The listing builds one solid part. Answer for the finished solid, in the listing's coordinates (mm). A direction names the side the tool comes from. Give positions to 0.01 mm unless a question says otherwise; leave off trailing zeros. Write each loop counter-clockwise with the first axis right and the second up, starting at its lowest first coordinate (ties: lowest second). Pieces come first, ordered by that corner, then holes. Notation, with made-up numbers: M 59.25,-9 L 93.25,-9 A5 cw 93.25,-4 Z; hole C 89.25,5.5 d8. An arc over 180 degrees is marked long. Answer as a JSON object with one key per item and string values.
```python
from build123d import *

# Parameters (mm, degrees)
SKETCH1_R           = 26.25
BOSS_EXTRUDE1_DEPTH = 133.5
SKETCH3_R           = 26.25
CUT_EXTRUDE1_DEPTH  = 232.63225164
CUT_EXTRUDE2_START  = -210
CUT_EXTRUDE2_DEPTH  = 105
FILLET1_R           = 20


with BuildPart() as part:
    # Sketch1 → Boss-Extrude1 (new body)
    with BuildSketch(Plane.XY):
        with BuildLine():
            Line((-52.5, 0), (-52.5, -157.5))
            Line((-52.5, -157.5), (52.5, -157.5))
            Line((52.5, -157.5), (52.5, 0))
            ThreePointArc((52.5, 0), (0, 52.5), (-52.5, 0))
        make_face()
        Circle(SKETCH1_R, mode=Mode.SUBTRACT)
    extrude(amount=BOSS_EXTRUDE1_DEPTH)

    # Sketch3 → Cut-Extrude1 (cut, through all)
    with BuildSketch(Plane.ZY.offset(52.5)):
        with Locations(Location((66.75, -105, 0), (0, 0, 270))):
            Circle(SKETCH3_R)
    extrude(amount=-CUT_EXTRUDE1_DEPTH, mode=Mode.SUBTRACT)

    # Sketch6 → Cut-Extrude2 (cut)
    with BuildSketch(Plane.XZ.offset(157.5).offset(CUT_EXTRUDE2_START)):
        Polygon((-52.5, 66.75), (-52.5, 44.5), (52.5, 44.5), (52.5, 89), (-52.5, 89), align=None)
    extrude(amount=CUT_EXTRUDE2_DEPTH, mode=Mode.SUBTRACT)

    # Fillet1
    fillet1_edges = [part.edges().sort_by_distance(p)[0] for p in [
        (0, -157.5, 133.5),
        (0, -157.5, 0),
    ]]
    fillet(fillet1_edges, radius=FILLET1_R)


solid = part.part
```
1. A cutting plane is placed at D-D, the plane z = 29. Give the vertices of the cut face in (x, y).
Verdict:
{"outline": "M -52.5,-157.5 L 52.5,-157.5 L 52.5,0 A52.5 ccw -52.5,0 Z; hole C 0,0 d52.5"}
2. A flat-ended cylindrical pin translates along its axis: pin 1 (6 mm diameter, centred on x = 19.5, z = 83, fed in from +Y). Find the tip coordinate at first contact, or state that the pin passes through.
Verdict:
{"pin 1": "stops at y = -52.5"}
3. The mould has two halves that part along Y. Classify faces 3 (the cylindrical face through (-1, -84, 51)), 4 (the cylindrical face through (0.735, -151.486, 127.797)), 5 (the flat face through (-1, -52.5, 67)): released by +Y, released by -Y, zero draft, split by the parting line, or undercut.
Verdict:
{"face 3": "undercut", "face 4": "released by -Y", "face 5": "released by +Y"}
4. A cutting plane is placed at B-B, the plane y = -105. Give the vertices of the cut face in (x, z), plus the area to 4 significant figures.
Verdict:
{"outline": "M -52.5,0 L 52.5,0 L 52.5,40.5 L -52.5,40.5 Z; M -52.5,93 L 52.5,93 L 52.5,133.5 L -52.5,133.5 Z", "area": "8,505 mm2"}
5. Consider line 1 along Y through (x, z) = (0, 105); line 2 along Z through (x, y) = (24, -39); line 3 along Z through (x, y) = (-29, -105). Determine where each line is inside the solid, lowest interval first.
Verdict:
{"line 1": "y = -157.5 to -26.25, 26.25 to 52.5", "line 2": "z = 0 to 44.5, 89 to 133.5", "line 3": "z = 0 to 40.5, 93 to 133.5"}
6. A cutting plane is placed at C-C, the plane z = 60. Give the vertices of the cut face in (x, y), plus the area to 3 significant figures.
Verdict:
{"outline": "M -52.5,-157.5 L 52.5,-157.5 L 52.5,-130.37 L -52.5,-130.37 Z; M -52.5,-79.63 L 52.5,-79.63 L 52.5,-52.5 L -52.5,-52.5 Z", "area": "5,700 mm2"}
7. For faces 1 (the cylindrical face through (0.735, -151.797, 6.014)), 2 (the flat face through (24, -11, 89)), determine the directions among +Z, -Z, +X, -X, +Y, -Y from which every point of the face is accessible in a straight line to the end or side of a thin tool.
Verdict:
{"face 1": "-Z, +X, -X, -Y", "face 2": "+X, -X, +Y"}
8. A cutting plane is placed at A-A, the plane x = 0. Give the vertices of the cut face in (y, z), plus the area to 3 significant figures.
Verdict:
{"outline": "M -157.5,20 A20 ccw -137.5,0 L -26.25,0 L -26.25,44.5 L -52.5,44.5 L -52.5,89 L -26.25,89 L -26.25,133.5 L -137.5,133.5 A20 ccw -157.5,113.5 Z; M 26.25,0 L 52.5,0 L 52.5,44.5 L 26.25,44.5 Z; M 26.25,89 L 52.5,89 L 52.5,133.5 L 26.25,133.5 Z; hole C -105,66.75 d52.5", "area": "16,400 mm2"}
